from build123d import *

# Parameters (mm, degrees)
BOSS_EXTRUDE1_DEPTH     = 11.1125
F_3_8_CLEARANCE_HOLE1_D = 10.0838
FILLET1_R               = 10
FILLET2_R               = 5
FILLET3_R               = 1.5
CUT_EXTRUDE1_REACH      = 1431.512
FILLET4_R               = 1


with BuildPart() as part:
    # Sketch4 → Boss-Extrude1 (new, symmetric)
    with BuildSketch(Plane(origin=(839.854692927, 426.912410879, 0), x_dir=(0, 0, -1), z_dir=(0.89140236631763, 0.4532127770962882, 0))):
        Polygon((-1293.587379373, 459.074586593), (-1293.587379373, 480.074586593), (-1263.587379373, 480.074586593), (-1225.891521519, 579.235261263), (-1225.891521519, 599.235261263), (-1203.425314933, 599.235261263), (-1203.425314933, 579.235261263), (-1249.104307407, 459.074586593), align=None)
    extrude(amount=BOSS_EXTRUDE1_DEPTH, both=True)

    # 3/8 Clearance Hole1 (through all)
    with Locations(Plane(origin=(0, 0, 1203.425314933), x_dir=(-1, 0, 0), z_dir=(0, 0, -1))):
        with Locations((-572.805743807, 952.158117087)):
            Hole(F_3_8_CLEARANCE_HOLE1_D / 2)

    # Fillet1
    fillet1_edges = [part.edges().sort_by_distance(p)[0] for p in [
        (577.337871578, 943.244093424, 1225.891521519),
        (577.337871578, 943.244093424, 1203.425314933),
    ]]
    fillet(fillet1_edges, radius=FILLET1_R)

    # Fillet2
    fillet2_edges = [part.edges().sort_by_distance(p)[0] for p in [
        (622.278756323, 854.852033377, 1263.587379373),
        (631.796224642, 836.132583685, 1249.104307407),
    ]]
    fillet(fillet2_edges, radius=FILLET2_R)

    # Fillet3
    fillet3_edges = [part.edges().sort_by_distance(p)[0] for p in [
        (568.273616036, 961.07214075, 1225.891521519),
        (568.273616036, 961.07214075, 1203.425314933),
    ]]
    fillet(fillet3_edges, radius=FILLET3_R)

    # Sketch9 → Cut-Extrude1 (cut, up to next)
    with BuildSketch(Plane(origin=(849.723172799, 432.02196164, 0), x_dir=(0, 0, -1), z_dir=(0.8914023663176289, 0.4532127770962904, 1.344287086354073e-15)), mode=Mode.PRIVATE) as cut_extrude1_sk1:
        with BuildLine():
            Line((-1220.891521519, 580.989746958), (-1208.425314933, 580.989746958))
            ThreePointArc((-1208.425314933, 580.989746958), (-1208.507569969, 580.086539083), (-1208.751628719, 579.213048567))
            Line((-1208.751628719, 579.213048567), (-1252.552657875, 463.992442123))
            Line((-1252.552657875, 463.992442123), (-1288.587379373, 463.992442123))
            Line((-1288.587379373, 463.992442123), (-1288.587379373, 474.992442123))
            Line((-1288.587379373, 474.992442123), (-1267.035729841, 474.992442123))
            ThreePointArc((-1267.035729841, 474.992442123), (-1261.358317042, 476.760371671), (-1257.688357413, 481.43904534))
            Line((-1257.688357413, 481.43904534), (-1221.870462877, 575.659651784))
            ThreePointArc((-1221.870462877, 575.659651784), (-1221.138286626, 578.280123334), (-1220.891521519, 580.989746958))
        make_face()
    cut_extrude1_tool1 = extrude(cut_extrude1_sk1.sketch, amount=-CUT_EXTRUDE1_REACH, mode=Mode.PRIVATE) & part.part
    add(cut_extrude1_tool1.solids().sort_by_distance((617.145834, 889.467119, 1243.085905))[0], mode=Mode.SUBTRACT)

    # Fillet4
    fillet4_edges = [part.edges().sort_by_distance(p)[0] for p in [
        (576.50548732, 944.8812699, 1208.425314933),
        (629.530160757, 840.589595516, 1288.587379373),
        (624.544820209, 850.395021546, 1288.587379373),
        (576.50548732, 944.8812699, 1220.891521519),
    ]]
    fillet(fillet4_edges, radius=FILLET4_R)


solid = part.part
Check sheet for the modelled part. Datum: model origin and axes. Units: mm. A direction names the side the tool comes from. Round coordinates to 2 decimals unless told otherwise and drop trailing zeros. Write each loop counter-clockwise with the first axis right and the second up, starting at its lowest first coordinate (ties: lowest second). Pieces come first, ordered by that corner, then holes. Notation, with made-up numbers: (-0.75, 55) - (56.25, 55) arc R18 ccw to (56.25, 84) - close; hole circle Ø5 at (14, -8). An arc over 180 degrees is marked (long way). Return JSON: item names as keys, results as strings.
Q1. Draft check along Y on faces 5 (the flat face through (599.905, 899.202, 1244.704)), 6 (the flat face through (603.194, 892.733, 1230.346)), 7 (the flat face through (631.93, 836.2, 1272.78)). Enter one of: released by +Y, released by -Y, zero draft, split by the parting line, or undercut.
Returned:
{"face 5": "released by +Y", "face 6": "undercut", "face 7": "released by -Y"}
Q2. Scan lines: L1, parallel to Z at x = 617.5, y = 854; L2, parallel to Z at x = 598, y = 905.5; L3, parallel to X at y = 941, z = 1215. Record each from-to range of solid material in increasing order. Write a range as from..to.
Returned:
{"L1": "z = 1240.59..1245.94, 1257.7..1263.56", "L2": "z = 1219.78..1225.12, 1236.89..1242.24", "L3": "x = 566.01..568.87"}
Q3. Depth check by flat-ended pin: P1, Ø9, axis at x = 623, y = 843, coming from the -Z side; P2, Ø3, axis at x = 618, z = 1276.5, coming from the -Y side; P3, Ø4, axis at x = 600, y = 923.5, coming from the -Z side. Enter the tip coordinate at first touch or a pass-through.
Returned:
{"P1": "stops at z = 1243.55", "P2": "stops at y = 846.3", "P3": "stops at z = 1213.26"}
Q4. Cross-section at C-C (z = 1282.5). Record the boundary of the cut face in (x, y), then the cut area to 3 significant figures.
Returned:
{"outline": "(612.37, 849.82) - (614.64, 845.36) - (634.45, 855.43) - (632.18, 859.89) - close; (619.62, 835.55) - (621.89, 831.1) - (641.7, 841.17) - (639.44, 845.63) - close", "area": "222 mm²"}
Q5. Cross-section at A-A (z = 1215.5). Record the boundary of the cut face in (x, y), then the cut area to 3 significant figures.
Returned:
{"outline": "(558.37, 956.04) - (566.6, 939.84) - (586.41, 949.92) - (578.18, 966.11) - close; (575.45, 922.44) - (581.83, 909.89) - (601.64, 919.97) - (595.26, 932.51) - close; hole circle Ø10.08 at (572.81, 952.16)", "area": "637 mm²"}
Q6. Access from +Z, -Z, +X, -X, +Y, -Y to the whole of each face (thin tool, end or side, straight path). Record for faces 1 (the flat face through (627, 846, 1288.587)), 2 (the flat face through (600.71, 897.62, 1240.03)), 3 (the cylindrical face through (631.55, 836.97, 1249.75)), 4 (the flat face through (576.5, 956.2, 1225.892)).
Returned:
{"face 1": "none", "face 2": "+X", "face 3": "-Z, +X, -Y", "face 4": "+Z, -X, +Y"}
Q7. Cross-section at B-B (y = 865). Record the boundary of the cut face in (x, z).
Returned:
{"outline": "(604.65, 1234.65) - (629.59, 1238.94) - (629.59, 1244.29) - (604.65, 1239.99) - close; (604.65, 1251.76) - (629.59, 1256.06) - (629.59, 1261.41) - (604.65, 1257.11) - close"}
